For this review, take the finished solid that the model builds, in its own axes (mm). A direction names the side the tool comes from. Round coordinates to 2 decimals unless told otherwise and drop trailing zeros. Order: outer loops, then holes, each group sorted by start corner. A loop starts at its lowest first (then second) coordinate and runs counter-clockwise, first axis right, second up. Notation, with made-up numbers: (58.25, -38.75) - (90.25, -38.75) arc R24 ccw to (90.25, -23.75) - close; hole circle Ø4 at (8, 22.5). An arc over 180 degrees is marked (long way). One line per question, with ' | ' between items.
Autodesk Inventor part; units mm, degrees
ref_plane "IP_1_XY" through (4.5, 0, 0) normal (1, 0, 0) x (0, 0, -1)
ref_plane "IP_1_YZ" through (4.5, 0, 0) normal (0, 0, -1) x (0, 1, 0)
ref_plane "IP_1_ZX" through (4.5, 0, 0) normal (0, 1, 0) x (1, 0, 0)
sketch "Sketch_1" plane through (0, 0, 0) normal (0, 0, 1) x (1, 0, 0)
  line L0 (8.3, 0) -> (0.7, 0)
  line L1 (0.7, 3.375) -> (8.3, 3.375)
  line L2 (8.3, 3.375) -> (8.3, 4.125)
  line L3 (8.3, 4.125) -> (0.7, 4.125)
  line L4 (0.7, 4.125) -> (0.7, 3.375)
revolve "Revolution1" add sketch "Sketch_1" angle 360 about axis through (8.3, 0, 0) along (1, 0, 0)
sketch "Sketch_2" plane through (0, 0, 0) normal (0, 0, 1) x (1, 0, 0)
  line L0 (7, 3.75) -> (2, 3.75)
  line L1 (2, 3.75) -> (2, 4.5)
  line L2 (2, 4.5) -> (7, 4.5)
  line L3 (7, 4.5) -> (7, 3.75)
  line L4 (7, 3.75) -> (2, 3.75)
revolve "Revolution2" cut sketch "Sketch_2" angle 360 about axis through (7, 3.75, 0) along (1, 0, 0)
pattern_circular "Circular Pattern1" count 9 over 360 about axis through (4.5, 0, 0) along (1, 0, 0) of "Revolution2"
ref_plane "IP_1_XY" through (4.5, 0, 0) normal (1, 0, 0) x (0, 0, -1)
ref_plane "IP_1_YZ" through (4.5, 0, 0) normal (0, 0, -1) x (0, 1, 0)
ref_plane "IP_1_ZX" through (4.5, 0, 0) normal (0, 1, 0) x (1, 0, 0)
ref_plane "IP_3_1_XY" through (4.5, 3.75, 0) normal (1, 0, 0) x (0, 0, -1)
ref_plane "IP_3_1_YZ" through (4.5, 3.75, 0) normal (0, 0, -1) x (0, 1, 0)
ref_plane "IP_3_1_ZX" through (4.5, 3.75, 0) normal (0, 1, 0) x (1, 0, 0)
ref_plane "IP_3_2_XY" through (4.5, 2.8727, 2.4105) normal (1, 0, 0) x (0, 0, -1)
ref_plane "IP_3_2_YZ" through (4.5, 2.8727, 2.4105) normal (0, 0, -1) x (0, 1, 0)
ref_plane "IP_3_2_ZX" through (4.5, 2.8727, 2.4105) normal (0, 1, 0) x (1, 0, 0)
ref_plane "IP_3_3_XY" through (4.5, 0.6512, 3.693) normal (1, 0, 0) x (0, 0, -1)
ref_plane "IP_3_3_YZ" through (4.5, 0.6512, 3.693) normal (0, 0, -1) x (0, 1, 0)
ref_plane "IP_3_3_ZX" through (4.5, 0.6512, 3.693) normal (0, 1, 0) x (1, 0, 0)
ref_plane "IP_3_4_XY" through (4.5, -1.875, 3.2476) normal (1, 0, 0) x (0, 0, -1)
ref_plane "IP_3_4_YZ" through (4.5, -1.875, 3.2476) normal (0, 0, -1) x (0, 1, 0)
ref_plane "IP_3_4_ZX" through (4.5, -1.875, 3.2476) normal (0, 1, 0) x (1, 0, 0)
ref_plane "IP_3_5_XY" through (4.5, -3.5238, 1.2826) normal (1, 0, 0) x (0, 0, -1)
ref_plane "IP_3_5_YZ" through (4.5, -3.5238, 1.2826) normal (0, 0, -1) x (0, 1, 0)
ref_plane "IP_3_5_ZX" through (4.5, -3.5238, 1.2826) normal (0, 1, 0) x (1, 0, 0)
ref_plane "IP_3_6_XY" through (4.5, -3.5238, -1.2826) normal (1, 0, 0) x (0, 0, -1)
ref_plane "IP_3_6_YZ" through (4.5, -3.5238, -1.2826) normal (0, 0, -1) x (0, 1, 0)
ref_plane "IP_3_6_ZX" through (4.5, -3.5238, -1.2826) normal (0, 1, 0) x (1, 0, 0)
ref_plane "IP_3_7_XY" through (4.5, -1.875, -3.2476) normal (1, 0, 0) x (0, 0, -1)
ref_plane "IP_3_7_YZ" through (4.5, -1.875, -3.2476) normal (0, 0, -1) x (0, 1, 0)
ref_plane "IP_3_7_ZX" through (4.5, -1.875, -3.2476) normal (0, 1, 0) x (1, 0, 0)
ref_plane "IP_3_8_XY" through (4.5, 0.6512, -3.693) normal (1, 0, 0) x (0, 0, -1)
ref_plane "IP_3_8_YZ" through (4.5, 0.6512, -3.693) normal (0, 0, -1) x (0, 1, 0)
ref_plane "IP_3_8_ZX" through (4.5, 0.6512, -3.693) normal (0, 1, 0) x (1, 0, 0)
ref_plane "IP_3_9_XY" through (4.5, 2.8727, -2.4105) normal (1, 0, 0) x (0, 0, -1)
ref_plane "IP_3_9_YZ" through (4.5, 2.8727, -2.4105) normal (0, 0, -1) x (0, 1, 0)
ref_plane "IP_3_9_ZX" through (4.5, 2.8727, -2.4105) normal (0, 1, 0) x (1, 0, 0)
properties part number "HK0609FMCA"
(1) Insertion check: pin 1 (1 mm diameter, centred on x = 4.5, y = 2.5, fed in from -Z). The pin has a flat end and moves straight along its axis. Give the tip position at first contact, or say it passes through.
Output values:
pin 1: z = -3.61
(2) We need section A-A on z = 0. State the section outline as (x, y) points (3 decimals).
Output values:
outline: (0.7, -4.125) - (8.3, -4.125) - (8.3, -3.375) - (0.7, -3.375) - close; (0.7, 3.375) - (2, 3.375) - (2, 4.125) - (0.7, 4.125) - close; (7, 3.375) - (8.3, 3.375) - (8.3, 4.125) - (7, 4.125) - close
(3) We need section B-B on x = 7.75. State the section outline as (y, z) points (3 decimals), plus the area to 3 significant figures.
Output values:
outline: circle Ø8.25 at (0, 0); hole circle Ø6.75 at (0, 0) | area: 17.7 mm^2
(4) For faces 3 (the cylindrical face through (4.6, -0.7, -3.3)), 4 (the flat face through (7, -3.5, -1.3)), list the 3-axis set-ups (+Z, -Z, +X, -X, +Y, -Y) from which the entire face can be reached by the end or side of a thin tool; tool diameter is ignored.
Output values:
face 3: +X, -X | face 4: none
(5) We need section D-D on z = 3.5. State the section outline as (x, y) points, plus the area to 3 significant figures.
Output values:
outline: (0.7, -2.18) - (2, -2.18) - (2, -1.17) - (7, -1.17) - (7, -2.18) - (8.3, -2.18) - (8.3, 2.18) - (0.7, 2.18) - close; hole (2, -0.07) - (7, -0.07) - (7, 1.38) - (2, 1.38) - close | area: 20.9 mm^2
(6) For probe 1 along X at (y, z) = (-2.5, -3); probe 2 along Z at (x, y) = (8.25, -2.5); probe 3 along Z at (x, y) = (1.25, 1.25), list the stretches that pass through material, from the lowest coordinate up. Write a range as [from, to].
Output values:
probe 1: [0.7, 2], [7, 8.3] | probe 2: [-3.28, -2.27], [2.27, 3.28] | probe 3: [-3.93, -3.13], [3.13, 3.93]
(7) We need section C-C on y = -0.25. State the section outline as (x, z) points.
Output values:
outline: (0.7, -4.12) - (8.3, -4.12) - (8.3, -3.37) - (0.7, -3.37) - close; (0.7, 3.37) - (8.3, 3.37) - (8.3, 4.12) - (0.7, 4.12) - close
(8) Mouldability with a two-part tool opening along X and no side actions: class faces 1 (the flat face through (7, 0.6, 3.7)), 2 (the flat face through (0.7, -2, -3)) as released by +X, released by -X, zero draft, split by the parting line, or undercut.
Output values:
face 1: undercut | face 2: released by -X
